```python
from build123d import *

# Parameters (mm, degrees)
BOSS_EXTRUDE1_DEPTH = 8
BOSS_EXTRUDE1_DRAFT = -10
SHELL1_T            = -1


with BuildPart() as part:
    # Sketch1 → Boss-Extrude1 (with draft: the straight prism first)
    with BuildSketch(Plane.XY):
        with BuildLine():
            ThreePointArc((0, -12.5), (12.5, 0), (0, 12.5))
            Line((0, 12.5), (-30, 12.5))
            ThreePointArc((-30, 12.5), (-42.5, 0), (-30, -12.5))
            Line((-30, -12.5), (0, -12.5))
        make_face()
    extrude(amount=BOSS_EXTRUDE1_DEPTH)
    # Boss-Extrude1: the draft: its side faces are tilted about the plane it starts from
    boss_extrude1_sides = [part.faces().sort_by_distance(p)[0] for p in [
        (-15, -12.5, 4),
        (12.5, 0, 4),
        (-15, 12.5, 4),
        (-42.5, 0, 4),
    ]]
    draft(boss_extrude1_sides, Plane.XY, BOSS_EXTRUDE1_DRAFT)

    # Shell1
    shell1_openings = [part.faces().sort_by_distance(p)[0] for p in [
        (-15, 0, 8),
    ]]
    offset(amount=SHELL1_T, openings=shell1_openings, kind=Kind.INTERSECTION)


solid = part.part
```
Geometry: final body of the model. Coordinates: model frame, mm. A direction names the side the tool comes from. Coordinates: 2 decimals unless noted, no trailing zeros. Order: outer loops, then holes, each group sorted by start corner. A loop starts at its lowest first (then second) coordinate and runs counter-clockwise, first axis right, second up. Notation, with made-up numbers: (79.25, -2.5) - (133.25, -2.5) arc R37 cw to (133.25, 35.5) - close; hole circle Ø10 at (-31.75, 63). An arc over 180 degrees is marked (long way). Write each question's results on one line, items separated by ' | '.
(1) Line query: line 1 (Y direction, x = -37.5, z = 5.25); line 2 (Y direction, x = -8, z = 5); line 3 (X direction, y = 2.75, z = 7). Output: solid intervals per line, ascending. Write a range as [from, to].
Values found:
line 1: y = [-11.14, -9.89], [9.89, 11.14] | line 2: y = [-13.38, -12.37], [12.37, 13.38] | line 3: x = [-43.46, -42.42], [12.42, 13.46]
(2) Section query B-B, the plane y = 0. Return the cut outline in (x, z), plus the area to 3 significant figures.
Values found:
outline: (-43.91, 8) - (-42.5, 0) - (12.5, 0) - (13.91, 8) - (12.9, 8) - (11.66, 1) - (-41.66, 1) - (-42.9, 8) - close | area: 69.4 mm²
(3) Set-up query: faces 1 (the face through (-15, 0, 1)), 2 (the face through (-43.036, 0.287, 3.055)). Return all of +Z, -Z, +X, -X, +Y, -Y with unobstructed straight access to the full face (end or side cutting, diameter ignored); none if empty.
Values found:
face 1: +Z | face 2: -Z, -X
(4) Section query A-A, the plane x = -9. Return the cut outline in (y, z), plus the area to 3 significant figures.
Values found:
outline: (-13.91, 8) - (-12.5, 0) - (12.5, 0) - (13.91, 8) - (12.9, 8) - (11.66, 1) - (-11.66, 1) - (-12.9, 8) - close | area: 39.4 mm²
(5) First-contact query: pin 1 Ø1 at (x, z) = (-23.5, 2.5) entering from +Y; pin 2 Ø3 at (y, z) = (-10.5, 1) entering from -X; pin 3 Ø1.5 at (y, z) = (-5, 6.5) entering from +X. Flat tips, straight axial feed; report the tip coordinate or a pass-through.
Values found:
pin 1: stops at y = 13.03 | pin 2: stops at x = -38.97 | pin 3: stops at x = 13
(6) Section query C-C, the plane z = 4.5. Return the cut outline in (x, y).
Values found:
outline: (-30, -13.29) - (0, -13.29) arc R13.29 ccw to (0, 13.29) - (-30, 13.29) arc R13.29 ccw to start; hole (-30, -12.28) - (0, -12.28) arc R12.28 ccw to (0, 12.28) - (-30, 12.28) arc R12.28 ccw to start
